The listing builds one solid part. Answer for the finished solid, in the listing's coordinates (mm). A direction names the side the tool comes from. Coordinates: 2 decimals unless noted, no trailing zeros. Write each loop counter-clockwise with the first axis right and the second up, starting at its lowest first coordinate (ties: lowest second). Pieces come first, ordered by that corner, then holes.
(1) The part is cut by section D-D on y = 0. Determine the outline of the cut face in (x, z), plus the area to 3 significant figures.
(2) Given P1, Ø5.5, axis at x = 1.5, y = -5.5, coming from the +Z side; P2, Ø3.5, axis at x = 7.5, z = 8, coming from the +Y side; P3, Ø9, axis at x = -9, z = 8, coming from the -Y side; P4, Ø2.5, axis at x = -9, z = 7, coming from the +Y side, each flat-ended and moving along its own axis, determine where each tip first touches the part or whether it passes through.
(3) The part is cut by section A-A on z = 16.75. Determine the outline of the cut face in (x, y), plus the area to 3 significant figures.
(4) Which of the six approach directions +Z, -Z, +X, -X, +Y, -Y give full straight-line access (tool end or side, diameter ignored) to faces 1 (the flat face through (-0.1, 4.5, 13)), 2 (the cylindrical face through (5.125, -10.331, 19.07)), 3 (the flat face through (8, 0, 10)), 4 (the flat face through (-11, 0.85, 6))?
(5) Straight lines are drawn through the part: line 1 (Y direction, x = 0.25, z = 19); line 2 (Y direction, x = 0, z = 3.75); line 3 (Z direction, x = -9, y = 6.75). For each, find the intervals that lie inside material, in ascending order.
(6) The part is cut by section C-C on z = 13.5. Determine the outline of the cut face in (x, y), plus the area to 3 significant figures.
(7) The part is cut by section B-B on x = 0. Determine the outline of the cut face in (y, z).
(8) For a pull along Z with two mould halves and no side action, classify faces 5 (the flat face through (-9, -7, 14)), 6 (the cylindrical face through (0, -4, 7)), 7 (the flat face through (-11, 4, 9)) as +Z half, -Z half, draft (parallel to the pull), parting line (faces both ways), or undercut.
from build123d import *

# Parameters (mm, degrees)
SKETCH1_R               = 15
BOSS_EXTRUDE1_DEPTH     = 25
CUT_EXTRUDE1_DEPTH      = 11
SKETCH4_R               = 4
CUT_EXTRUDE2_DEPTH      = 14
SKETCH5_R               = 8
CUT_EXTRUDE3_DEPTH      = 1
SKETCH6_W               = 28.841933153
SKETCH6_H               = 1.7
CUT_EXTRUDE4_DEPTH      = 14
SKETCH7_W               = 7.091355734
SKETCH7_H               = 1.7
BOSS_EXTRUDE2_DEPTH     = 2
CHAMFER1_SIZE           = 11
CUT_EXTRUDE5_DEPTH      = 14
CUT_EXTRUDE5_DEPTH_BACK = 14
SKETCH8_R               = 2
SKETCH9_R               = 3.75
CUT_EXTRUDE6_DEPTH      = 11
FILLET1_R               = 2
FILLET2_R               = 1


with BuildPart() as part:
    # Sketch1 → Boss-Extrude1 (new body)
    with BuildSketch(Plane.XY):
        Circle(SKETCH1_R)
    extrude(amount=BOSS_EXTRUDE1_DEPTH)

    # Sketch3 → Cut-Extrude1 (cut)
    with BuildSketch(Plane.XY.offset(25)):
        with BuildLine():
            ThreePointArc((2.96875, -7.428763251), (31, 0), (2.96875, 7.428763251))
            ThreePointArc((2.96875, 7.428763251), (0, 8), (-2.96875, 7.428763251))
            ThreePointArc((-2.96875, 7.428763251), (-31, 0), (-2.96875, -7.428763251))
            ThreePointArc((-2.96875, -7.428763251), (0, -8), (2.96875, -7.428763251))
        make_face()
    extrude(amount=-CUT_EXTRUDE1_DEPTH, mode=Mode.SUBTRACT)

    # Sketch4 → Cut-Extrude2 (cut)
    with BuildSketch(Plane.XY.offset(14)):
        Circle(SKETCH4_R)
    extrude(amount=-CUT_EXTRUDE2_DEPTH, mode=Mode.SUBTRACT)

    # Sketch5 → Cut-Extrude3 (cut)
    with BuildSketch(Plane.XY.offset(14)):
        Circle(SKETCH5_R)
    extrude(amount=-CUT_EXTRUDE3_DEPTH, mode=Mode.SUBTRACT)

    # Sketch6 → Cut-Extrude4 (cut)
    with BuildSketch(Plane.XY.offset(14)):
        with Locations((-3.420966576, 0)):
            Rectangle(SKETCH6_W, SKETCH6_H)
    extrude(amount=-CUT_EXTRUDE4_DEPTH, mode=Mode.SUBTRACT)

    # Sketch7 → Boss-Extrude2 (add)
    with BuildSketch(Plane(origin=(0, 0, 0), x_dir=(-1, 0, 0), z_dir=(0, 0, -1))):
        with Locations((-7.454322133, 0)):
            Rectangle(SKETCH7_W, SKETCH7_H)
    extrude(amount=-BOSS_EXTRUDE2_DEPTH)

    # Chamfer1
    # the kernel refuses this chamfer: 11 mm, written as the material it adds along each edge
    with BuildSketch(Plane(origin=(11, -0.85, 2), x_dir=(0.027495876610586414, 0, 0.9996219169112968), z_dir=(0, 1, 0))) as chamfer1_piece_1_section:
        Polygon((CHAMFER1_SIZE * 0.999621916911, -CHAMFER1_SIZE * 0.0274958766106), (-CHAMFER1_SIZE * 0.0274958766106, -CHAMFER1_SIZE * 0.999621916911), (0, 0), align=None)
    chamfer1_piece_1 = extrude(amount=1.7, mode=Mode.PRIVATE)
    chamfer1_piece_1 = split(chamfer1_piece_1, bisect_by=Plane(origin=(3.908644266, 0, 6.042844173), z_dir=(1, 0, 0)), keep=Keep.TOP, mode=Mode.PRIVATE)
    add(chamfer1_piece_1)

    # Sketch8 → Cut-Extrude5 (cut, two sides: drawn at the far end of the back side and taken through both)
    with BuildSketch(Plane(origin=(0, 0, 0), x_dir=(1, 0, 0), z_dir=(0, 1, 0)).offset(-CUT_EXTRUDE5_DEPTH_BACK)):
        with Locations(Location((-9, -7, 0), (0, 0, 90))):
            Circle(SKETCH8_R)
    extrude(amount=CUT_EXTRUDE5_DEPTH + CUT_EXTRUDE5_DEPTH_BACK, mode=Mode.SUBTRACT)

    # Sketch9 → Cut-Extrude6 (cut)
    with BuildSketch(Plane(origin=(0, 15, 0), x_dir=(1, 0, 0), z_dir=(0, 1, 0))):
        with Locations(Location((-9, -7, 0), (0, 0, 270))):
            Circle(SKETCH9_R)
    extrude(amount=-CUT_EXTRUDE6_DEPTH, mode=Mode.SUBTRACT)

    # Fillet1
    fillet1_edges = [part.edges().sort_by_distance(p)[0] for p in [
        (15, 0, 0),
    ]]
    fillet(fillet1_edges, radius=FILLET1_R)

    # Fillet2
    fillet2_edges = [part.edges().sort_by_distance(p)[0] for p in [
        (-5.160499055, 10.368472369, 25),
        (0, -8, 25),
        (5.160499055, -10.368472369, 25),
        (0, 8, 25),
        (-5.160499055, -10.368472369, 25),
        (5.160499055, 10.368472369, 25),
    ]]
    fillet(fillet2_edges, radius=FILLET2_R)


solid = part.part
Model answer:
1. outline: (3.91, 0) - (13, 0) arc R2 ccw to (15, 2) - (15, 14) - (11, 14) - (11, 13) - (3.91, 5.91) - close
1. area: 122 mm2
2. P1: stops at z = 24.84
2. P2: stops at y = 13.85
2. P3: stops at y = -14.31
2. P4: passes through
3. outline: (-8, -12.69) arc R15 ccw to (8, -12.69) arc R15 cw to (2.97, -7.43) arc R8 cw to (-2.97, -7.43) arc R15 cw to start; (-8, 12.69) arc R15 cw to (-2.97, 7.43) arc R8 cw to (2.97, 7.43) arc R15 cw to (8, 12.69) arc R15 ccw to start
3. area: 152 mm2
4. face 1: +Z
4. face 2: +Z, +X
4. face 3: +Z, -X
4. face 4: +Z, -Z, -X
5. line 1: y = -15 to -8, 8 to 15
5. line 2: y = -15 to -4, 4 to 15
5. line 3: z = 0 to 3.25, 10.75 to 14
6. outline: (-14.98, -0.85) arc R15 ccw (long way) to (-14.98, 0.85) - (-7.95, 0.85) arc R8 cw to (7.95, 0.85) - (11, 0.85) - (11, -0.85) - (7.95, -0.85) arc R8 cw to (-7.95, -0.85) - close
6. area: 489 mm2
7. outline: (-15, 2) arc R2 ccw to (-13, 0) - (-4, 0) - (-4, 13) - (-8, 13) - (-8, 24) arc R1 ccw to (-9, 25) - (-15, 25) - close; (4, 0) - (13, 0) arc R2 ccw to (15, 2) - (15, 25) - (9, 25) arc R1 ccw to (8, 24) - (8, 13) - (4, 13) - close
8. face 5: +Z half
8. face 6: draft
8. face 7: undercut
